from build123d import *

# Parameters (mm, degrees)
SKETCH2_R           = 7
BOSS_EXTRUDE1_DEPTH = 22


with BuildPart() as part:
    # Sketch2 → Boss-Extrude1 (new, symmetric)
    with BuildSketch(Plane(origin=(0, 0, 0), x_dir=(1, 0, 0), z_dir=(0, 1, 0))):
        with BuildLine():
            Line((-8.044825261, -3.211346175), (-8.044825261, 14.788653825))
            Line((-8.044825261, 14.788653825), (-1.044825261, 21.788653825))
            Line((-1.044825261, 21.788653825), (5.955174739, 21.788653825))
            Line((5.955174739, 21.788653825), (28.316555575, 17.845739058))
            ThreePointArc((28.316555575, 17.845739058), (40.516273445, 19.770697967), (48.955174739, 28.788653825))
            Line((48.955174739, 28.788653825), (72.955174739, 28.788653825))
            Line((72.955174739, 28.788653825), (77.955174739, 23.788653825))
            Line((77.955174739, 23.788653825), (77.955174739, 4.788653825))
            Line((77.955174739, 4.788653825), (48.955174739, -29.211346175))
            Line((48.955174739, -29.211346175), (43.252154792, -29.211346175))
            ThreePointArc((43.252154792, -29.211346175), (38.813182595, -22.327018236), (36.476352392, -14.476052057))
            ThreePointArc((36.476352392, -14.476052057), (34.795949432, -11.424759943), (31.530713651, -10.211346175))
            Line((31.530713651, -10.211346175), (-1.044825261, -10.211346175))
            Line((-1.044825261, -10.211346175), (-8.044825261, -3.211346175))
        make_face()
        with Locations(Location((5.955174739, 3.788653825, 0), (0, 0, 270))):
            Circle(SKETCH2_R, mode=Mode.SUBTRACT)
    extrude(amount=BOSS_EXTRUDE1_DEPTH, both=True)


solid = part.part
The model under review builds one solid part; all positions refer to its coordinate system, in mm. A direction names the side the tool comes from. Coordinates: 2 decimals unless noted, no trailing zeros. Write each loop counter-clockwise with the first axis right and the second up, starting at its lowest first coordinate (ties: lowest second). Pieces come first, ordered by that corner, then holes. Notation, with made-up numbers: (32, 46.5) - (62, 46.5) arc R14 ccw to (62, 51.5) - close; hole circle Ø5 at (35, 12.5). An arc over 180 degrees is marked (long way). Answer as a JSON object with one key per item and string values. Group by question number.
1. Add section B-B (z = -7). Give the boundary of the cut face in (x, y).
2. Machinability: for faces 4 (the face through (16.979, 0.308, -19.845)), 5 (the face through (36, -22, -7)), 6 (the face through (75.42, 0.308, -26.324)), 7 (the face through (2, 0, -21.789)), 8 (the face through (15, 0, 10.211)), which of the approach directions +Z, -Z, +X, -X, +Y, -Y give a long, thin tool a straight path to every point of the face, cutting with its end or side? Answer none if there is none.
3. Add section D-D (x = 32.5). Give the boundary of the cut face in (y, z).
4. Add section A-A (y = 19.5). Give the boundary of the cut face in (x, z), plus the area to 3 significant figures.
5. Add section C-C (z = 0.5). Give the boundary of the cut face in (x, y), plus the area to 3 significant figures.
6. Clearance check with flat-ended pins moving along their axes: pin 1 Ø2 at (x, y) = (1.5, -5.5) entering from -Z; pin 2 Ø1.5 at (x, y) = (32, -4) entering from +Z; pin 3 Ø6 at (y, z) = (-2, 4) entering from +X. State where each tip first meets the part, or that it passes through.
7. To check wall thickness, follow probe 1 along Z at (x, y) = (0.5, -4.5); probe 2 along X at (y, z) = (17.5, -7.5); probe 3 along X at (y, z) = (-14, -9.5). State the ranges of each line that lie inside material, in increasing order.
8. Mouldability with a two-part tool opening along X and no side actions: class faces 1 (the face through (40.36, 0.31, -19.69)), 2 (the face through (77.955, 0, -14)), 3 (the face through (36, 22, -7)) as pulls with the +X half, pulls with the -X half, needs draft (parallel to the pull), parting line crosses it, or undercut.
Findings:
{
 "1": {"outline": "(-8.04, -22) - (-0.26, -22) - (-0.26, 22) - (-8.04, 22) - close; (12.18, -22) - (77.96, -22) - (77.96, 22) - (12.18, 22) - close"},
 "2": {"face 4": "-Z, +Y, -Y", "face 5": "+Z, -Z, +X, -X, -Y", "face 6": "-Z, +X, +Y, -Y", "face 7": "-Z, -X, +Y, -Y", "face 8": "+Z, -X, +Y, -Y"},
 "3": {"outline": "(-22, -17.58) - (22, -17.58) - (22, 10.31) - (-22, 10.31) - close"},
 "4": {"outline": "(-8.04, -14.79) - (-1.04, -21.79) - (5.96, -21.79) - (28.32, -17.85) arc R19 cw to (48.96, -28.79) - (72.96, -28.79) - (77.96, -23.79) - (77.96, -4.79) - (48.96, 29.21) - (43.25, 29.21) arc R29 ccw to (36.48, 14.48) arc R5 cw to (31.53, 10.21) - (-1.04, 10.21) - (-8.04, 3.21) - close; hole circle Ø14 at (5.96, -3.79)", "area": "2,930 mm²"},
 "5": {"outline": "(-8.04, -22) - (0.42, -22) - (0.42, 22) - (-8.04, 22) - close; (11.49, -22) - (73.44, -22) - (73.44, 22) - (11.49, 22) - close", "area": "3,100 mm²"},
 "6": {"pin 1": "z = -21.79", "pin 2": "z = 10.36", "pin 3": "x = 73.02"},
 "7": {"probe 1": "-21.79 to -8.18, 0.6 to 10.21", "probe 2": "-8.04 to 0.02, 11.89 to 77.96", "probe 3": "-8.04 to 1.91, 10 to 77.96"},
 "8": {"face 1": "undercut", "face 2": "pulls with the +X half", "face 3": "needs draft"}
}
